Could you check a few things on this model? Use its own coordinates, in mm. Round coordinates to 2 decimals unless told otherwise and drop trailing zeros. Loops run counter-clockwise (first coordinate to the right, second up) from the corner with the lowest first, then second, coordinate; pieces in that order, holes last. Notation, with made-up numbers: M -28,26 L 16,26 A11 ccw 16,32 Z; hole C 44.25,74 d7. An arc over 180 degrees is marked long. Answer in a Markdown table with one row per item.
```python
from build123d import *

# Parameters (mm, degrees)
SKETCH_1_W           = 45
SKETCH_1_H           = 68
EXTRUDE_1_DEPTH      = 10
FILLET_1_R           = 5
SKETCH_2_R           = 1.5
EXTRUDE_2_DEPTH      = 1.4
SKETCH_3_OUTSIDE_W   = 63.662
SKETCH_3_OUTSIDE_H   = 28.662
SKETCH_3_OUTSIDE_W_2 = 45
SKETCH_3_OUTSIDE_H_2 = 10
SKETCH_3_OUTSIDE_R   = 2.5
CUT_EXTRUDE_1_DEPTH  = 5


with BuildPart() as part:
    # 草图1 → 凸台-拉伸1 (new body)
    with BuildSketch(Plane.XY):
        Rectangle(SKETCH_1_W, SKETCH_1_H)
    extrude(amount=EXTRUDE_1_DEPTH)

    # 圆角1
    fillet_1_edges = [part.edges().sort_by_distance(p)[0] for p in [
        (22.5, 34, 5),
    ]]
    fillet(fillet_1_edges, radius=FILLET_1_R)

    # 草图2 → 凸台-拉伸2 (add)
    with BuildSketch(Plane(origin=(0, 34, 0), x_dir=(1, 0, 0), z_dir=(0, 1, 0))):
        with Locations(Location((-18.5, -5, 0), (0, 0, 90))):
            Circle(SKETCH_2_R)
    extrude(amount=EXTRUDE_2_DEPTH)

    # 草图3 outside → 切除-拉伸1 (cut)
    # profile 1 of 2: a face of its own
    with BuildSketch(Plane.XZ.offset(34)):
        with Locations((0, 5)):
            Rectangle(SKETCH_3_OUTSIDE_W, SKETCH_3_OUTSIDE_H)
        with Locations((0, 5)):
            Rectangle(SKETCH_3_OUTSIDE_W_2, SKETCH_3_OUTSIDE_H_2, mode=Mode.SUBTRACT)
    # profile 2 of 2: a face of its own
    with BuildSketch(Plane.XZ.offset(34)):
        with Locations(Location((-18.5, 5, 0), (0, 0, 270))):
            Circle(SKETCH_3_OUTSIDE_R)
    extrude(amount=-CUT_EXTRUDE_1_DEPTH, mode=Mode.SUBTRACT)


solid = part.part
```
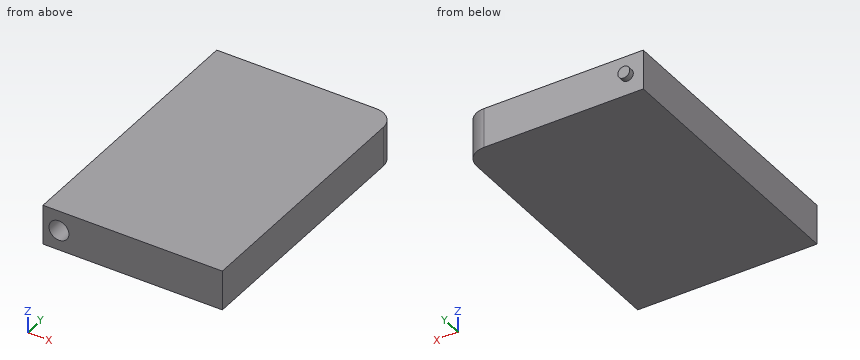
1) I want a section at C-C, the plane z = 9. Please give me the cut outline in (x, y).
Computed:
| item | result |
|---|---|
| outline | M -22.5,-34 L 22.5,-34 L 22.5,29 A5 ccw 17.5,34 L -22.5,34 Z |
2) I want a section at A-A, the plane z = 5. Please give me the cut outline in (x, y).
Computed:
| item | result |
|---|---|
| outline | M -22.5,-34 L -21,-34 L -21,-29 L -16,-29 L -16,-34 L 22.5,-34 L 22.5,29 A5 ccw 17.5,34 L -17,34 L -17,35.4 L -20,35.4 L -20,34 L -22.5,34 Z |
3) I want a section at B-B, the plane x = -18.5. Please give me the cut outline in (y, z).
Computed:
| item | result |
|---|---|
| outline | M -34,0 L 34,0 L 34,3.5 L 35.4,3.5 L 35.4,6.5 L 34,6.5 L 34,10 L -34,10 L -34,7.5 L -29,7.5 L -29,2.5 L -34,2.5 Z |
4) I need wall thicknesses on line 1 (X direction, y = -30.5, z = 5); line 2 (Y direction, x = -19.5, z = 0.75); line 3 (Z direction, x = -18, y = -30). Which ranges of each line are inside material? Lowest first, please.
Computed:
| item | result |
|---|---|
| line 1 | x = -22.5 to -21, -16 to 22.5 |
| line 2 | y = -34 to 34 |
| line 3 | z = 0 to 2.55, 7.45 to 10 |
5) I want a section at D-D, the plane x = -5. Please give me the cut outline in (y, z).
Computed:
| item | result |
|---|---|
| outline | M -34,0 L 34,0 L 34,10 L -34,10 Z |
